Verification items for the finished model (mm, model axes). Face numbers are marked on the shaded views. Give positions to 0.01 mm unless a question says otherwise; leave off trailing zeros. Write each loop counter-clockwise with the first axis right and the second up, starting at its lowest first coordinate (ties: lowest second). Pieces come first, ordered by that corner, then holes. Notation, with made-up numbers: (32.5, 62) -> (52.5, 62) arc R15 ccw to (52.5, 80) -> close; hole circle Ø3 at (78.25, 63). An arc over 180 degrees is marked (long way). Use CSV: the item, a comma, the result in double quotes. Start each with the question number.
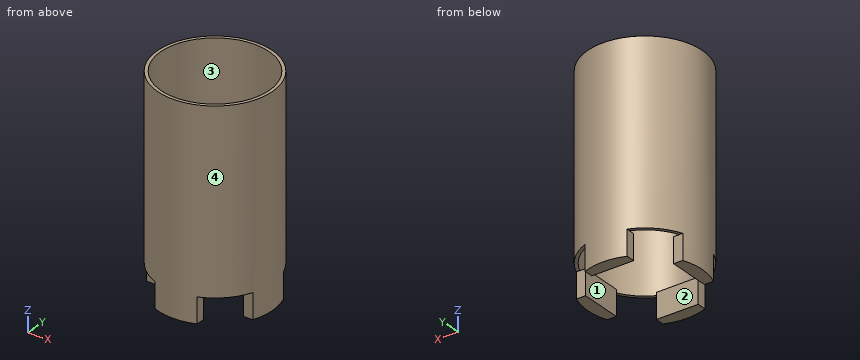
```python
from build123d import *

# Parameters (mm, degrees)
F0_R     = 27.25
F0_R_2   = 25.75
F1_DEPTH = 85
F2_W     = 20
F2_H     = 17.491485
F2_W_2   = 14.608384
F2_H_2   = 20
F3_DEPTH = 12
F4_R     = 27.25
F5_DEPTH = 100


with BuildPart() as f1:
    # F0 (on Top) → F1 (new body)
    with BuildSketch(Plane.XY):
        Circle(F0_R)
        Circle(F0_R_2, mode=Mode.SUBTRACT)
    extrude(amount=F1_DEPTH)

    # F2 (on Top) → F3 (join)
    with BuildSketch(Plane.XY):
        with Locations((0, -29.745742)):
            Rectangle(F2_W, F2_H)
        with Locations((-28.304192, 0)):
            Rectangle(F2_W_2, F2_H_2)
        with Locations((0, 29.745742)):
            Rectangle(F2_W, F2_H)
        with Locations((28.304192, 0)):
            Rectangle(F2_W_2, F2_H_2)
    extrude(amount=-F3_DEPTH)

    # F4 (on face) → F5 (intersect, symmetric)
    with BuildSketch(Plane(origin=(0, 0, 0), x_dir=(1, 0, 0), z_dir=(0, 0, -1))):
        Circle(F4_R)
    extrude(amount=F5_DEPTH, both=True, mode=Mode.INTERSECT)


solid = f1.part
```
(1) Section check D-D on y = -22. Record the cut outline in (x, z).
(2) Go/stop test with flat-tipped pins: pin 1 (8 mm diameter, centred on x = 15, y = 12.5, fed in from +Z); pin 2 (1 mm diameter, centred on x = 14.5, z = 7, fed in from -Y); pin 3 (7.5 mm diameter, centred on x = -15, y = -18, fed in from -Z); pin 4 (1.5 mm diameter, centred on y = -3, z = 53, fed in from +X). Record where each tip stops, or that it passes through.
(3) Section check C-C on z = 5. Record the cut outline in (x, y).
(4) Draft check along X on the marked faces 1, 2, 3 and 4. Enter one of: released by +X, released by -X, zero draft, split by the parting line, or undercut.
(5) Section check A-A on y = 0. Record the cut outline in (x, z), then the cut area to 3 significant figures.
(6) Thickness scan on line 1 (X direction, y = 0, z = 27); line 2 (X direction, y = 14.5, z = 68). Record the ranges inside material, lowest first. Write a range as from..to.
Data:
1,outline,"(-16.08, 0) -> (-13.38, 0) -> (-13.38, 85) -> (-16.08, 85) -> close; (-10, -12) -> (10, -12) -> (10, 0) -> (-10, 0) -> close; (13.38, 0) -> (16.08, 0) -> (16.08, 85) -> (13.38, 85) -> close"
2,pin 1,"passes through"
2,pin 2,"stops at y = -23.38"
2,pin 3,"stops at z = 0"
2,pin 4,"stops at x = 27.16"
3,outline,"circle Ø54.5 at (0, 0); hole circle Ø51.5 at (0, 0)"
4,face 1,"undercut"
4,face 2,"zero draft"
4,face 3,"undercut"
4,face 4,"split by the parting line"
5,outline,"(-27.25, -12) -> (-21, -12) -> (-21, 0) -> (-25.75, 0) -> (-25.75, 85) -> (-27.25, 85) -> close; (21, -12) -> (27.25, -12) -> (27.25, 85) -> (25.75, 85) -> (25.75, 0) -> (21, 0) -> close"
5,area,"405 mm2"
6,line 1,"x = -27.25..-25.75, 25.75..27.25"
6,line 2,"x = -23.07..-21.28, 21.28..23.07"
